The listing builds one solid part. Answer for the finished solid, in the listing's coordinates (mm). Face numbers are marked on the shaded views. A direction names the side the tool comes from. Give positions to 0.01 mm unless a question says otherwise; leave off trailing zeros. Write each loop counter-clockwise with the first axis right and the second up, starting at its lowest first coordinate (ties: lowest second). Pieces come first, ordered by that corner, then holes. Notation, with made-up numbers: M 56,24.5 L 113,24.5 A25 cw 113,49.5 Z; hole C -20,87.5 d1. An arc over 180 degrees is marked long. Answer as a JSON object with one key per item and string values.
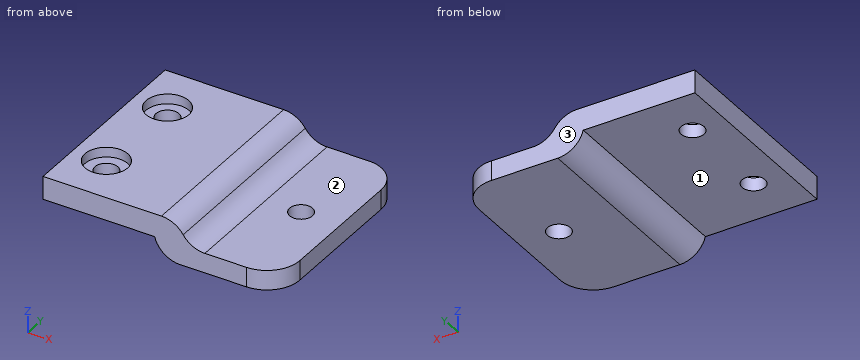
```python
from build123d import *

# Parameters (mm, degrees)
F0_W        = 5
F0_H        = 30
F0_W_2      = 17
F0_R        = 1.75
F1_DEPTH    = 3.5
F2_DEPTH    = 3
F3_T1_DEPTH = 49.843134833
F3_T3_DEPTH = 49.364916731
F4_R        = 3.25
F5_DEPTH    = 1.5
F6_R        = 4


# Not quite as in the source:
# - a fillet or chamfer that OpenCascade refuses, or shapes differently, is made with other operations: its cross-section is extruded or revolved along the edge and cut away or added


with BuildPart() as f1:
    # F0 (on Top) → F1 (new body)
    with BuildSketch(Plane.XY):
        Rectangle(F0_W, F0_H)
        with Locations((-11, 0)):
            Rectangle(F0_W_2, F0_H)
        with Locations((-14.5, -7.5)):
            Circle(F0_R, mode=Mode.SUBTRACT)
        with Locations((-14.5, 7.5)):
            Circle(F0_R, mode=Mode.SUBTRACT)
    extrude(amount=F1_DEPTH)

    # F0 (on Top) → F2 (join)
    with BuildSketch(Plane.XY):
        with BuildLine():
            Line((11.5, 15), (2.5, 15))
            Line((2.5, 15), (2.5, -15))
            Line((2.5, -15), (11.5, -15))
            ThreePointArc((11.5, -15), (15.0355339059, -13.5355339059), (16.5, -10))
            Line((16.5, -10), (16.5, 10))
            ThreePointArc((16.5, 10), (15.0355339059, 13.5355339059), (11.5, 15))
        make_face()
        with Locations((10.5, 0)):
            Circle(F0_R, mode=Mode.SUBTRACT)
        Rectangle(F0_W, F0_H)
    extrude(amount=-F2_DEPTH)

    # F3: fillet of radius 4 on 2 edges, made by hand

    # F3_s2 → F3_t1 (cut)
    with BuildSketch(Plane.XZ.offset(-24.9215674165)):
        with BuildLine():
            ThreePointArc((2.5, 0), (1.1771243445, 2.5), (-1.4686269666, 3.5))
            Line((-1.4686269666, 3.5), (2.5, 3.5))
            Line((2.5, 3.5), (2.5, 0))
        make_face()
    extrude(amount=F3_T1_DEPTH, mode=Mode.SUBTRACT)

    # F3_s4 → F3_t3 (cut)
    with BuildSketch(Plane.XZ.offset(-24.6824583655)):
        with BuildLine():
            ThreePointArc((-2.5, 0), (-1.0765063966, -2.1622776602), (1.3729833462, -3))
            Line((1.3729833462, -3), (-2.5, -3))
            Line((-2.5, -3), (-2.5, 0))
        make_face()
    extrude(amount=F3_T3_DEPTH, mode=Mode.SUBTRACT)

    # F4 (on face) → F5 (cut)
    with BuildSketch(Plane.XY.offset(3.5)):
        with Locations((-14.5, 7.5)):
            Circle(F4_R)
        with Locations((-14.5, -7.5)):
            Circle(F4_R)
    extrude(amount=-F5_DEPTH, mode=Mode.SUBTRACT)

    # F6
    f6_edges = [f1.edges().sort_by_distance(p)[0] for p in [
        (2.5, 0, 0),
    ]]
    fillet(f6_edges, radius=F6_R)


solid = f1.part
```
1. Consider line 1 along Y through (x, z) = (-14.5, 1.6); line 2 along Y through (x, z) = (-14.5, 3.1); line 3 along Y through (x, z) = (10.5, -2). Determine where each line is inside the solid, lowest interval first.
Verdict:
{"line 1": "y = -15 to -9.25, -5.75 to 5.75, 9.25 to 15", "line 2": "y = -15 to -10.75, -4.25 to 4.25, 10.75 to 15", "line 3": "y = -15 to -1.75, 1.75 to 15"}
2. For the marked faces 1, 2 and 3, determine the directions among +Z, -Z, +X, -X, +Y, -Y from which every point of the face is accessible in a straight line to the end or side of a thin tool.
Verdict:
{"face 1": "-Z, -X, +Y, -Y", "face 2": "+Z, +X, +Y, -Y", "face 3": "+Z, -Z, +X, -X, +Y"}
3. A cutting plane is placed at A-A, the plane y = 0. Give the vertices of the cut face in (x, z).
Verdict:
{"outline": "M -19.5,0 L -2.5,0 A4 ccw 1.37,-3 L 8.75,-3 L 8.75,0 L 5.15,0 A4 cw 1.84,1.75 A4 ccw -1.47,3.5 L -19.5,3.5 Z; M 12.25,-3 L 16.5,-3 L 16.5,0 L 12.25,0 Z"}
4. A cutting plane is placed at D-D, the plane z = -1.75. Give the vertices of the cut face in (x, y), plus the area to 3 significant figures.
Verdict:
{"outline": "M -1.53,-15 L 11.5,-15 A5 ccw 16.5,-10 L 16.5,10 A5 ccw 11.5,15 L -1.53,15 Z; hole C 10.5,0 d3.5", "area": "521 mm2"}
5. A cutting plane is placed at C-C, the plane x = 11. Give the vertices of the cut face in (y, z).
Verdict:
{"outline": "M -15,-3 L -1.68,-3 L -1.68,0 L -15,0 Z; M 1.68,-3 L 15,-3 L 15,0 L 1.68,0 Z"}
6. Flat-ended cylindrical pins translate along their axes: pin 1 (1.5 mm diameter, centred on x = 7, y = -3, fed in from +Z); pin 2 (2 mm diameter, centred on x = 10.5, y = 0, fed in from -Z); pin 3 (1.5 mm diameter, centred on x = 0, y = 2.5, fed in from -Z); pin 4 (5.5 mm diameter, centred on x = -14.5, y = -7.5, fed in from -Z). Find the tip coordinate at first contact, or state that the pin passes through.
Verdict:
{"pin 1": "stops at z = 0", "pin 2": "passes through", "pin 3": "stops at z = -2.95", "pin 4": "stops at z = 0"}
7. A cutting plane is placed at B-B, the plane x = -14. Give the vertices of the cut face in (y, z), plus the area to 3 significant figures.
Verdict:
{"outline": "M -15,0 L -9.18,0 L -9.18,2 L -10.71,2 L -10.71,3.5 L -15,3.5 Z; M -5.82,0 L 5.82,0 L 5.82,2 L 4.29,2 L 4.29,3.5 L -4.29,3.5 L -4.29,2 L -5.82,2 Z; M 9.18,0 L 15,0 L 15,3.5 L 10.71,3.5 L 10.71,2 L 9.18,2 Z", "area": "72.3 mm2"}
